from build123d import *

# Parameters (mm, degrees)
ESQUISSE1_W             = 65
ESQUISSE1_H             = 150
BOSS_EXTRU_1_DEPTH      = 60
ESQUISSE2_W             = 145
ESQUISSE2_H             = 50
ENL_V_MAT_EXTRU_1_DEPTH = 4


with BuildPart() as part:
    # Esquisse1 → Boss.-Extru.1 (new body)
    with BuildSketch(Plane(origin=(0, 0, 0), x_dir=(1, 0, 0), z_dir=(0, 1, 0))):
        Rectangle(ESQUISSE1_W, ESQUISSE1_H)
    extrude(amount=BOSS_EXTRU_1_DEPTH)

    # Esquisse2 → Enlèv. mat.-Extru.1 (cut)
    with BuildSketch(Plane.ZY.offset(32.5)):
        with Locations((2.5, 30)):
            Rectangle(ESQUISSE2_W, ESQUISSE2_H)
    enl_v_mat_extru_1 = extrude(amount=-ENL_V_MAT_EXTRU_1_DEPTH, mode=Mode.SUBTRACT)

    # Symétrie1: Enlèv. mat.-Extru.1 across plane
    add(enl_v_mat_extru_1.mirror(Plane(origin=(0, 0, 0), x_dir=(0, 0, 1), z_dir=(1, 0, 0))), mode=Mode.SUBTRACT)


solid = part.part
Work out the finished part from the listing and answer in its coordinate system (mm). A direction names the side the tool comes from. Round coordinates to 2 decimals unless told otherwise and drop trailing zeros. Loops run counter-clockwise (first coordinate to the right, second up) from the corner with the lowest first, then second, coordinate; pieces in that order, holes last. Notation, with made-up numbers: M 28,48 L 39,48 A20 ccw 39,68 Z; hole C 84.5,60 d10. An arc over 180 degrees is marked long. One line per question, with ' | ' between items. Start each with the question number.
(1) A tool of negligible diameter and unlimited length cuts with its end or side. For faces 4 (the face through (-31, 5, 1)), 5 (the face through (32.5, 57, -11)), 6 (the face through (31, 5, 1)), from which of +Z, -Z, +X, -X, +Y, -Y can it reach the whole face along a straight path? Write none if from no direction.
(2) A cutting plane is placed at A-A on y = 17.5. Write down the section's boundary in (x, z).
(3) For a pull along Y with two mould halves and no side action, classify faces 1 (the face through (31, 55, 1)), 2 (the face through (0, 60, -1)), 3 (the face through (0, 30, -75)) as released by +Y, released by -Y, zero draft, split by the parting line, or undercut.
(4) Find the intervals of material crossed by line 1 (X direction, y = 9, z = -61); line 2 (Z direction, x = -29.5, y = 11.5), in increasing order.
(5) A cutting plane is placed at B-B on z = -41.5. Write down the section's boundary in (x, y), plus the area to 3 significant figures.
(6) Flat-ended cylindrical pins translate along their axes: pin 1 Ø15 at (y, z) = (35.5, 31.5) entering from -X; pin 2 Ø1.2 at (x, y) = (30, 28.5) entering from +Z; pin 3 Ø3 at (y, z) = (40, -8) entering from +X. Find the tip coordinate at first contact, or state that the pin passes through.
Geometry check:
1) face 4: +Z, -X | face 5: +Z, -Z, +X, +Y, -Y | face 6: +Z, +X
2) outline: M -32.5,-75 L 32.5,-75 L 32.5,-70 L 28.5,-70 L 28.5,75 L -28.5,75 L -28.5,-70 L -32.5,-70 Z
3) face 1: undercut | face 2: released by +Y | face 3: zero draft
4) line 1: x = -28.5 to 28.5 | line 2: z = -75 to -70
5) outline: M -32.5,0 L 32.5,0 L 32.5,5 L 28.5,5 L 28.5,55 L 32.5,55 L 32.5,60 L -32.5,60 L -32.5,55 L -28.5,55 L -28.5,5 L -32.5,5 Z | area: 3,500 mm²
6) pin 1: stops at x = -28.5 | pin 2: stops at z = -70 | pin 3: stops at x = 28.5
